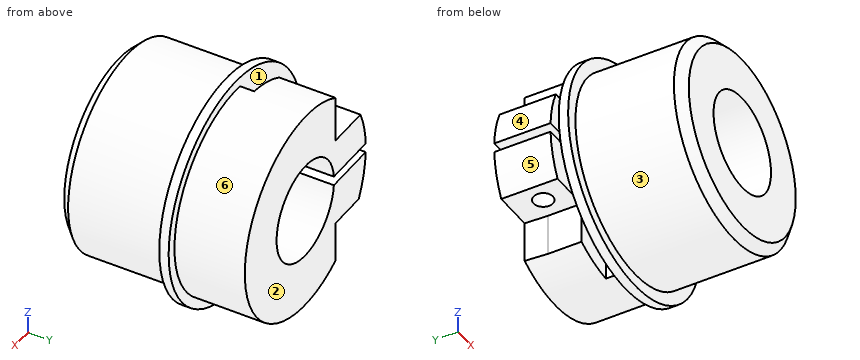
Autodesk Inventor part; units mm, degrees
ref_plane "YZ Plane" through (0, 0, 0) normal (1, 0, 0) x (0, 1, 0)
ref_plane "XZ Plane" through (0, 0, 0) normal (0, 1, 0) x (-1, 0, 0)
ref_plane "XY Plane" through (0, 0, 0) normal (0, 0, 1) x (1, 0, 0)
sketch "Sketch1" plane through (0, 0, 0) normal (0, 1, 0) x (-1, 0, 0)
  circle A0 centre (0, 0) radius 21.35
  dimension "d0" = 42.7
extrude "Extrusion1" add sketch "Sketch1" along normal blind 23
sketch "Sketch2" plane through (0, 23, 0) normal (0, 1, 0) x (1, 0, 0)
  circle A0 centre (0, 0) radius 24
  dimension "d3" = 48
extrude "Extrusion2" add sketch "Sketch2" along normal blind 2
sketch "Sketch3" plane through (0, 25, 0) normal (0, 1, 0) x (1, 0, 0)
  circle A0 centre (0, 0) radius 24
  circle A1 centre (0, 0) radius 21.9
  dimension "d6" = 43.8
extrude "Extrusion3" add sketch "Sketch3" along normal blind 15 contours A1
sketch "Sketch5" plane through (0, 40, 0) normal (0, 1, 0) x (1, 0, 0)
  line L0 (0, 0) -> (-16.9119, 0)
  line L1 (-16.9119, 0) -> (-16.9119, 11.9609)
  line L2 (-16.9119, 11.9609) -> (0, 11.9609)
  line L3 (0, 11.9609) -> (0, 0)
sketch "Sketch8" plane through (0, 40, 0) normal (0, 1, 0) x (1, 0, 0)
  circle A0 centre (0, 0) radius 10.4
  dimension "d18" = 20.8
extrude "Extrusion5" cut sketch "Sketch8" against normal through all
sketch "Sketch9" plane through (0, 40, 0) normal (0, 1, 0) x (1, 0, 0)
  arc A0 (-20.347, 8.1) -> (20.347, 8.1) centre (0, 0) ccw
  line L0 (-21.9, 0) -> (-10.9, 0)
  line L1 (-10.9, 0) -> (-10.9, -21.2976)
  line L2 (-10.9, -21.2976) -> (-22.7633, -21.2976)
  line L3 (-22.7633, -21.2976) -> (-22.7633, 0)
  line L4 (-22.7633, 0) -> (-21.9, 0)
  line L5 (-22.7633, 0) -> (-22.7633, 1)
  line L6 (-22.7633, 1) -> (-8.5921, 1)
  line L7 (-8.5921, 1) -> (-8.5921, -0.9996)
  line L8 (-8.5921, -0.9996) -> (-22.7633, -0.9996)
  line L9 (-10.9, -0.9996) -> (-10.9, -8.9996)
  line L10 (-10.9, -8.9996) -> (-22.7633, -8.9996)
  point P0 (-19.9654, -8.9996)
  point P1 (-10.9, -18.9947)
  dimension "d21" = 11
  dimension "d22" = 1
  dimension "d23" = 8
extrude "Extrusion6" cut sketch "Sketch9" against normal blind 15 contours L6 L7 L8 L1 L0 A0 | A0 L4 L5 L6 | L0 L1 L8 A0 | A0 L8 L3 L4 | L10 L1 A0
sketch "Sketch10" plane through (-19.9654, 40, 8.9996) normal (0, 0, 1) x (1, 0, 0)
  circle A0 centre (4.7692, -6.5146) radius 2.55
  point P0 (19.9654, -40)
  dimension "d26" = 5.1
hole "Hole1" at (-15.1962, 33.4854, 8.9996) direction (0, 0, -1) diameter 4.134 end through all
chamfer "Chamfer1" distance 2 angle 45 1 edges at (21.35, 0, 0)
ref_plane "Work Plane4" through (-21.8772, 40, -0.0002) normal (0, 0, 1) x (1, 0, 0)
ref_plane "Work Plane5" through (-21.8772, 40, 21.9998) normal (0, 0, 1) x (1, 0, 0)
sketch "Sketch11" plane through (-21.8772, 40, 21.9998) normal (0, 0, 1) x (1, 0, 0)
  line L0 (0, -15) -> (1.9118, -15)
  line L1 (0, -15) -> (0, -12)
  line L2 (0, 0) -> (0, -15)
  line L3 (0, -12) -> (20, -12)
  line L4 (20, -12) -> (20, -15)
  line L5 (20, -15) -> (0, -15)
  line L6 (45.8772, -15) -> (-2.1228, -15)
  point P0 (21.8772, -40)
  point P1 (10.9772, -15)
  dimension "d39" = 3
  dimension "d42" = 20
extrude "Extrusion7" cut sketch "Sketch11" against normal through all
ref_plane "Work Plane6" through (-21.8772, 40, -18.2502) normal (0, 0, 1) x (1, 0, 0)
sketch "Sketch13" plane through (-21.8772, 40, -18.2502) normal (0, 0, 1) x (1, 0, 0)
  line L0 (11.5253, 0) -> (11.5253, -12)
  line L1 (10.9772, 0) -> (11.5253, -12)
  line L2 (0, -12) -> (0, 0)
  line L3 (11.5253, -12) -> (0, -12)
  line L4 (0, -12) -> (0, 0)
  line L5 (0, 0) -> (11.201, 0)
  line L6 (1.9118, 0) -> (10.9772, 0)
  line L7 (11.201, 0) -> (11.201, -12)
  line L8 (11.5253, -12) -> (0, -12)
  point P0 (21.8772, -40)
  point P1 (11.201, -4.9004)
extrude "Extrusion9" cut sketch "Sketch13" along normal mid plane 16 contours L1 L7 L3 L2 L5
properties part number "Probe holder"
The listing builds one solid part. Answer for the finished solid, in the listing's coordinates (mm). Face numbers are marked on the shaded views. A direction names the side the tool comes from. Give positions to 0.01 mm unless a question says otherwise; leave off trailing zeros. Write each loop counter-clockwise with the first axis right and the second up, starting at its lowest first coordinate (ties: lowest second). Pieces come first, ordered by that corner, then holes. Notation, with made-up numbers: (1.5, 66.25) -> (18.5, 66.25) arc R30 ccw to (18.5, 102.25) -> close; hole circle Ø1 at (39.25, 12). An arc over 180 degrees is marked (long way). One line per question, with ' | ' between items. Start each with the question number.
1. Section A-A (z = 0) is taken. Determine the outline of the cut face in (x, y).
2. For a pull along Y with two mould halves and no side action, classify the marked faces 1, 2 and 3 as pulls with the +Y half, pulls with the -Y half, needs draft (parallel to the pull), parting line crosses it, or undercut.
3. Section B-B (x = 0) is taken. Determine the outline of the cut face in (y, z), plus the area to 3 significant figures.
4. For the marked faces 4, 5 and 6, determine the directions among +Z, -Z, +X, -X, +Y, -Y from which every point of the face is accessible in a straight line to the end or side of a thin tool.
5. Given pin 1 Ø1.5 at (x, y) = (2.5, 10) entering from -Z; pin 2 Ø9 at (x, y) = (-16.5, 35) entering from +Z; pin 3 Ø5 at (x, z) = (-11, 12) entering from +Y; pin 4 Ø6 at (x, y) = (-13.5, 7.5) entering from +Z, each flat-ended and moving along its own axis, determine where each tip first touches the part or whether it passes through.
6. Find the intervals of material crossed by probe 1 along Y at (x, z) = (-2, -11); probe 2 along Z at (x, y) = (0, 30); probe 3 along Y at (x, z) = (-15.5, -7), in increasing order.
7. Section C-C (z = -6) is taken. State how many separate pieces and enclosed holes the cut face has, plus the area to 3 significant figures.
8. Section D-D (y = 10.5) is taken. Determine the outline of the cut face in (x, z), plus the area to 3 significant figures.
Response values:
1) outline: (-24, 23) -> (-21.35, 23) -> (-21.35, 2) -> (-19.35, 0) -> (-10.4, 0) -> (-10.4, 25) -> (-24, 25) -> close; (10.4, 0) -> (19.35, 0) -> (21.35, 2) -> (21.35, 23) -> (24, 23) -> (24, 25) -> (21.9, 25) -> (21.9, 40) -> (10.4, 40) -> close
2) face 1: undercut | face 2: pulls with the +Y half | face 3: needs draft
3) outline: (0, -19.35) -> (2, -21.35) -> (23, -21.35) -> (23, -24) -> (25, -24) -> (25, -21.9) -> (40, -21.9) -> (40, -10.4) -> (0, -10.4) -> close; (0, 10.4) -> (40, 10.4) -> (40, 21.9) -> (25, 21.9) -> (25, 24) -> (23, 24) -> (23, 21.35) -> (2, 21.35) -> (0, 19.35) -> close | area: 899 mm2
4) face 4: +Z, -X, +Y | face 5: -Z, -X, +Y | face 6: +Y
5) pin 1: z = -21.28 | pin 2: z = 9 | pin 3: y = 40 | pin 4: z = 18.59
6) probe 1: 0 to 25, 28 to 40 | probe 2: -21.9 to -10.4, 10.4 to 21.9 | probe 3: 0 to 25, 28 to 31.44, 35.53 to 40
7) separate pieces: 3 | enclosed holes: 1 | area: 932 mm2
8) outline: circle Ø42.7 at (0, 0); hole circle Ø20.8 at (0, 0) | area: 1,090 mm2
